Part model, mm, in its own coordinate system. Face numbers are marked on the shaded views. Coordinates: 2 decimals unless noted, no trailing zeros. Order: outer loops, then holes, each group sorted by start corner. A loop starts at its lowest first (then second) coordinate and runs counter-clockwise, first axis right, second up. Notation, with made-up numbers: M 24,84 L 80,84 A9 cw 80,97 Z; hole C 23.25,-13 d1. An arc over 180 degrees is marked long. Answer in a Markdown table with one row per item. Add a question column.
from build123d import *

# Parameters (mm, degrees)
SKETCH_W        = 62.81
SKETCH_H        = 94.56
PAD_DEPTH       = 5.27
SKETCH001_W     = 51.3
SKETCH001_H     = 83.16
POCKET_DEPTH    = 3.27
SKETCH002_W     = 56.5
SKETCH002_H     = 90.5
POCKET001_DEPTH = 1.5
PAD001_DEPTH    = 90.5
PAD002_DEPTH    = 90.5
PAD003_DEPTH    = 28.5
SKETCH006_R     = 1.25
PAD004_DEPTH    = 16.5
PAD005_DEPTH    = 5.25


with BuildPart() as part:
    # Sketch → Pad (new body)
    with BuildSketch(Plane.XY):
        Rectangle(SKETCH_W, SKETCH_H)
    extrude(amount=PAD_DEPTH)

    # Sketch001 → Pocket (cut)
    with BuildSketch(Plane.XY.offset(5.27)):
        Rectangle(SKETCH001_W, SKETCH001_H)
    extrude(amount=-POCKET_DEPTH, mode=Mode.SUBTRACT)

    # Sketch002 → Pocket001 (cut)
    with BuildSketch(Plane.XY.offset(3.5)):
        with Locations((0, 2.03)):
            Rectangle(SKETCH002_W, SKETCH002_H)
    extrude(amount=-POCKET001_DEPTH, mode=Mode.SUBTRACT)

    # Sketch003 → Pad001 (join)
    with BuildSketch(Plane.XZ.offset(43.22)):
        Polygon((-25.65, 3.5), (-28.25, 2.2), (-28.25, 3.5), align=None)
    extrude(amount=-PAD001_DEPTH)

    # Sketch004 → Pad002 (join)
    with BuildSketch(Plane.XZ.offset(43.22)):
        Polygon((25.65, 3.5), (28.25, 3.5), (28.25, 2.2), align=None)
    extrude(amount=-PAD002_DEPTH)

    # Sketch005 → Pad003 (join, symmetric)
    with BuildSketch(Plane.YZ):
        Polygon((-41.58, 3.5), (-43.22, 2.293188), (-43.22, 3.5), align=None)
    extrude(amount=PAD003_DEPTH, both=True)

    # Sketch006 → Pad004 (join, symmetric)
    with BuildSketch(Plane.XZ):
        with BuildLine():
            Line((-28.615358, 0.722295), (-28.615358, -1.865583))
            ThreePointArc((-28.615358, -1.865583), (-26.115358, -4.365583), (-23.615358, -1.865583))
            Line((-23.615358, 0.722295), (-23.615358, -1.865583))
            Line((-28.615358, 0.722295), (-23.615358, 0.722295))
        make_face()
        with Locations((-26.115358, -1.865583)):
            Circle(SKETCH006_R, mode=Mode.SUBTRACT)
    pad004 = extrude(amount=PAD004_DEPTH, both=True)

    # Sketch007 → Pad005 (join)
    with BuildSketch(Plane.XY):
        with BuildLine():
            ThreePointArc((-10.054045, -51.641873), (0.400338, -69.077796), (9.629085, -50.963278))
            Line((9.629085, -50.963278), (6.442785, -46.244865))
            Line((-6.927812, -46.244865), (6.442785, -46.244865))
            Line((-6.927812, -46.244865), (-10.054045, -51.641873))
        make_face()
    extrude(amount=PAD005_DEPTH)

    # Mirrored: Pad004 across Sketch006 V_Axis
    add(pad004.mirror(Plane(origin=(0, 0, 0), x_dir=(0, -1, 0), z_dir=(1, 0, 0))))


solid = part.part
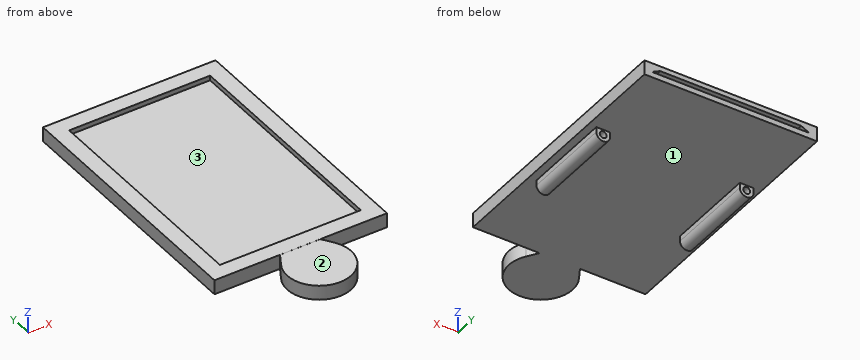
(1) Wall check: line 1 (Y direction, x = -22.5, z = 4); line 2 (X direction, y = -25.5, z = 4.5) (3 decimals); line 3 (Y direction, x = 10, z = 5). Give the ranges that are in metal, low to high.
(2) Pull direction X, two halves, no side cores. Call the marked faces 1, 2 and 3: pulls with the +X half, pulls with the -X half, needs draft (parallel to the pull), parting line crosses it, or undercut.
(3) Slice it at D-D (y = 35). List the corners of the cut face in (x, z) (3 decimals).
(4) Slice it at C-C (x = -21). List the corners of the cut face in (y, z).
(5) Drop flat-ended pins along their axis: P1, Ø3.5, axis at x = -25, z = -2, coming from the +Y side; P2, Ø8, axis at x = -21, y = -2, coming from the -Z side; P3, Ø1, axis at x = -23.5, y = -38.5, coming from the -Z side; P4, Ø1.5, axis at x = 26.12, z = -1.87, coming from the -Y side. Give the stop position or say it passes through.
(6) Slice it at B-B (y = 10). List the corners of the cut face in (x, z) (3 decimals).
Computed:
| question | item | result |
|---|---|---|
| 1 | line 1 | y = -47.28 to -41.58, 41.58 to 47.28 |
| 1 | line 2 | x = -31.405 to -25.65, 25.65 to 31.405 |
| 1 | line 3 | y = -63.38 to -51.55, -47.28 to -41.58, 41.58 to 47.28 |
| 2 | face 1 | undercut |
| 2 | face 2 | needs draft |
| 2 | face 3 | undercut |
| 3 | outline | M -31.405,0 L 31.405,0 L 31.405,5.27 L 25.65,5.27 L 25.65,3.5 L 28.25,2.2 L 28.25,2 L -28.25,2 L -28.25,2.2 L -25.65,3.5 L -25.65,5.27 L -31.405,5.27 Z |
| 4 | outline | M -47.28,0 L 47.28,0 L 47.28,2 L -43.22,2 L -43.22,2.29 L -41.58,3.5 L -41.58,5.27 L -47.28,5.27 Z; M 41.58,3.5 L 47.28,3.5 L 47.28,5.27 L 41.58,5.27 Z |
| 5 | P1 | stops at y = 16.5 |
| 5 | P2 | stops at z = -4.1 |
| 5 | P3 | stops at z = 0 |
| 5 | P4 | passes through |
| 6 | outline | M -31.405,0 L -28.615,0 L -28.615,-1.866 A2.5 ccw -23.615,-1.866 L -23.615,0 L 23.615,0 L 23.615,-1.866 A2.5 ccw 28.615,-1.866 L 28.615,0 L 31.405,0 L 31.405,5.27 L 25.65,5.27 L 25.65,3.5 L 28.25,2.2 L 28.25,2 L -28.25,2 L -28.25,2.2 L -25.65,3.5 L -25.65,5.27 L -31.405,5.27 Z; hole C -26.115,-1.866 d2.5; hole C 26.115,-1.866 d2.5 |
